Verification items for the finished model (mm, model axes). A direction names the side the tool comes from. Round coordinates to 2 decimals unless told otherwise and drop trailing zeros. Loops run counter-clockwise (first coordinate to the right, second up) from the corner with the lowest first, then second, coordinate; pieces in that order, holes last. Notation, with made-up numbers: (-5, -19) - (0, -19) arc R27 cw to (0, 3) - close; hole circle Ø3 at (48, 22.25). An arc over 180 degrees is marked (long way). Use CSV: the item, a comma, the result in double quotes.
```python
from build123d import *

# Parameters (mm, degrees)
SKETCH_1_R          = 6
SKETCH_1_R_2        = 2.55
EXTRUDE_1_DEPTH     = 7.5
SKETCH_2_R          = 1.5
CUT_EXTRUDE_1_DEPTH = 25.763884994
CUT_EXTRUDE_2_DEPTH = 9.5
FILLET_1_R          = 1


with BuildPart() as part:
    # 草图1 → 凸台-拉伸1 (new, symmetric)
    # profile 1 of 2: a face of its own
    with BuildSketch(Plane.XY):
        with Locations((0, 13)):
            Circle(SKETCH_1_R)
        with Locations((0, 13)):
            Circle(SKETCH_1_R_2, mode=Mode.SUBTRACT)
    # profile 2 of 2: a face of its own
    with BuildSketch(Plane.XY):
        with BuildLine():
            ThreePointArc((4.410490728, 8.932129361), (0, 7), (-4.410490728, 8.932129361))
            Line((-4.410490728, 8.932129361), (-6, 3))
            Line((-6, 3), (-14, 3))
            Line((-14, 3), (-14, 0))
            Line((-14, 0), (14, 0))
            Line((14, 0), (14, 3))
            Line((14, 3), (6, 3))
            Line((6, 3), (4.410490728, 8.932129361))
        make_face()
    extrude(amount=EXTRUDE_1_DEPTH, both=True)

    # 草图2 → 切除-拉伸1 (cut, through all)
    with BuildSketch(Plane.XZ):
        with Locations((-10, 4)):
            Circle(SKETCH_2_R)
        with Locations((-10, -4)):
            Circle(SKETCH_2_R)
        with Locations((10, -4)):
            Circle(SKETCH_2_R)
        with Locations(Location((10, 4, 0), (0, 0, 180))):
            Circle(SKETCH_2_R)
    extrude(amount=-CUT_EXTRUDE_1_DEPTH, mode=Mode.SUBTRACT)

    # 草图3 → 切除-拉伸2 (cut)
    with BuildSketch(Plane(origin=(0, 0, -7.5), x_dir=(-1, 0, 0), z_dir=(0, 0, -1))):
        Polygon((0, 8.150257739), (4.2, 10.575128869), (4.2, 15.424871131), (0, 17.849742261), (-4.2, 15.424871131), (-4.2, 10.575128869), align=None)
    extrude(amount=-CUT_EXTRUDE_2_DEPTH, mode=Mode.SUBTRACT)

    # 圆角1
    fillet_1_edges = [part.edges().sort_by_distance(p)[0] for p in [
        (4.410490728, 8.932129361, 0),
        (6, 3, 0),
        (-6, 3, 0),
        (-4.410490728, 8.932129361, 0),
        (0, 8.150257739, -2.75),
        (4.2, 10.575128869, -2.75),
        (4.2, 15.424871131, -2.75),
        (0, 17.849742261, -2.75),
        (-4.2, 15.424871131, -2.75),
        (-4.2, 10.575128869, -2.75),
    ]]
    fillet(fillet_1_edges, radius=FILLET_1_R)


solid = part.part
```
1) Cross-section at A-A, the plane z = 4. Record the cut outline in (x, y), then the cut area to 3 significant figures.
Returned:
outline,"(-14, 0) - (-11.5, 0) - (-11.5, 3) - (-14, 3) - close; (-8.5, 0) - (8.5, 0) - (8.5, 3) - (6.77, 3) arc R1 cw to (5.8, 3.74) - (4.55, 8.43) arc R1 cw to (4.72, 9.3) arc R6 ccw (long way) to (-4.72, 9.3) arc R1 cw to (-4.55, 8.43) - (-5.8, 3.74) arc R1 cw to (-6.77, 3) - (-8.5, 3) - close; (11.5, 0) - (14, 0) - (14, 3) - (11.5, 3) - close; hole circle Ø5.1 at (0, 13)"
area,"209 mm²"
2) Cross-section at C-C, the plane y = 13. Record the cut outline in (x, z), then the cut area to 4 significant figures.
Returned:
outline,"(-6, -7.5) - (-4.2, -7.5) - (-4.2, 2) - (-2.55, 2) - (-2.55, 7.5) - (-6, 7.5) - close; (2.55, 2) - (4.2, 2) - (4.2, -7.5) - (6, -7.5) - (6, 7.5) - (2.55, 7.5) - close"
area,"72.15 mm²"
3) Mould release check, pull along Y, two halves, no side actions. Record for faces 4 (the face through (-14, 2, 0)), 5 (the face through (4.07, 15.34, -2.68)), 6 (the face through (0, 0, 0)), 7 (the face through (-10, 3, 0)): +Y half, -Y half, draft (parallel to the pull), parting line (faces both ways), or undercut.
Returned:
face 4,"draft"
face 5,"undercut"
face 6,"-Y half"
face 7,"+Y half"
4) Cross-section at D-D, the plane x = 10. Record the cut outline in (y, z), then the cut area to 3 significant figures.
Returned:
outline,"(0, -7.5) - (3, -7.5) - (3, -5.5) - (0, -5.5) - close; (0, -2.5) - (3, -2.5) - (3, 2.5) - (0, 2.5) - close; (0, 5.5) - (3, 5.5) - (3, 7.5) - (0, 7.5) - close"
area,"27.0 mm²"
5) Thickness scan on probe 1 along Z at (x, y) = (-10, 0.8); probe 2 along Y at (x, z) = (0, 4.2); probe 3 along Z at (x, y) = (-11.25, 2.75). Record the ranges inside material, lowest first. Write a range as [from, to].
Returned:
probe 1,"z = [-7.5, -5.5], [-2.5, 2.5], [5.5, 7.5]"
probe 2,"y = [0, 10.45], [15.55, 19]"
probe 3,"z = [-7.5, -4.83], [-3.17, 3.17], [4.83, 7.5]"
6) Cross-section at B-B, the plane x = 0. Record the cut outline in (y, z).
Returned:
outline,"(0, -7.5) - (8.3, -7.5) - (8.3, 2) - (10.45, 2) - (10.45, 7.5) - (0, 7.5) - close; (15.55, 2) - (17.7, 2) - (17.7, -7.5) - (19, -7.5) - (19, 7.5) - (15.55, 7.5) - close"
7) Gauge pin test, flat ends, axial feed: pin 1 Ø3 at (y, z) = (13.5, -1) entering from +X; pin 2 Ø3 at (y, z) = (12, -2) entering from -X; pin 3 Ø2.5 at (x, y) = (-2, 14.5) entering from -Z. Record the tip position at first contact, or that the pin passes through.
Returned:
pin 1,"stops at x = 6"
pin 2,"stops at x = -6"
pin 3,"stops at z = 2"
8) Access from +Z, -Z, +X, -X, +Y, -Y to the whole of each face (thin tool, end or side, straight path). Record for faces 1 (the face through (-5.165, 6.117, 0.105)), 2 (the face through (2, 11, 2)), 3 (the face through (4.533, 8.891, -0.105)).
Returned:
face 1,"+Z, -Z, -X"
face 2,"-Z"
face 3,"+Z, -Z, +X"
